Can you work these out from the model? Positions are in its coordinate system, mm. Coordinates: 2 decimals unless noted, no trailing zeros. Order: outer loops, then holes, each group sorted by start corner. A loop starts at its lowest first (then second) coordinate and runs counter-clockwise, first axis right, second up. Notation, with made-up numbers: (67.5, 32.25) -> (74.5, 32.25) arc R21 ccw to (74.5, 62.25) -> close; hole circle Ø4 at (87.25, 51). An arc over 180 degrees is marked (long way). Answer in a Markdown table with one row per item. Add a question column.
1. Imagine slicing it at D-D on y = 2.7. Write out the boundary of the cut face in (x, z), plus the area to 3 significant figures.
2. Imagine slicing it at B-B on x = -11.5. Write out the boundary of the cut face in (y, z), plus the area to 3 significant figures.
3. Imagine slicing it at C-C on x = -5. Write out the boundary of the cut face in (y, z), plus the area to 3 significant figures.
4. If I drill on line 1 along Z through (x, y) = (17.5, 2.6); line 2 along Z through (x, y) = (-9, 0.85); line 3 along Y through (x, z) = (9.5, 12.75), over which ranges is the centre line in solid material (lowest first)? Write a range as [from, to].
5. Imagine slicing it at A-A on y = 1.1. Write out the boundary of the cut face in (x, z), plus the area to 3 significant figures.
6. Will this pin go through, and if not, where does the flat tip stop? pin 1 (2 mm diameter, centred on x = -1.5, z = 3.5, fed in from -Y).
from build123d import *

# Parameters (mm, degrees)
F0_W        = 36.83
F0_H        = 3.048
F1_DEPTH    = 13.97
F3_T1_DEPTH = 60.1094845304
F4_DEPTH    = 25.4


# Not quite as in the source:
# - a fillet or chamfer that OpenCascade refuses, or shapes differently, is made with other operations: its cross-section is extruded or revolved along the edge and cut away or added


with BuildPart() as f1:
    # F0 (on Top) → F1 (new body)
    with BuildSketch(Plane.XY):
        with Locations((-0.254, 1.524)):
            Rectangle(F0_W, F0_H)
    extrude(amount=F1_DEPTH)

    # F3: fillet of radius 5.08 on 1 edges, made by hand

    # F3_s2 → F3_t1 (cut)
    with BuildSketch(Plane.YZ.offset(-30.3087422652)):
        with BuildLine():
            ThreePointArc((3.048, 9.3141030939), (2.2182329348, 12.0965336861), (0, 13.97))
            Line((0, 13.97), (3.048, 13.97))
            Line((3.048, 13.97), (3.048, 9.3141030939))
        make_face()
    extrude(amount=F3_T1_DEPTH, mode=Mode.SUBTRACT)

    # F2 (on face) → F4 (cut)
    with BuildSketch(Plane.XZ):
        Polygon((-15.494, 12.5322954744), (-14.6639409051, 13.97), (-16.3240590949, 13.97), align=None)
        Polygon((-4.3572939367, 13.97), (-6.3107060633, 13.97), (-5.334, 12.2782954744), align=None)
        Polygon((5.6560590949, 13.97), (3.9959409051, 13.97), (4.826, 12.5322954744), align=None)
        Polygon((15.8160590949, 13.97), (14.1559409051, 13.97), (14.986, 12.5322954744), align=None)
    extrude(amount=-F4_DEPTH, mode=Mode.SUBTRACT)


solid = f1.part
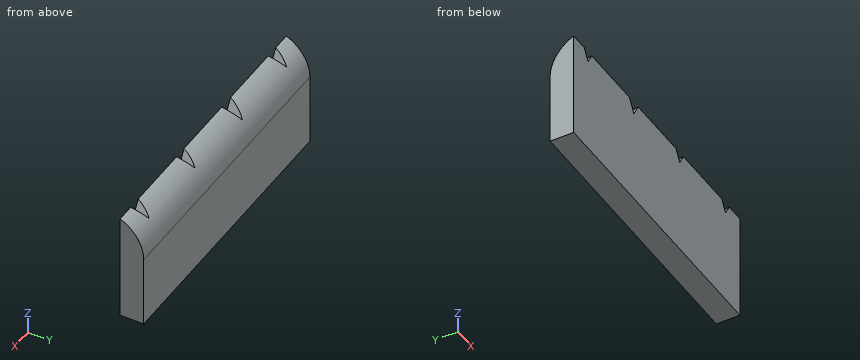
Answers follow:
| question | item | result |
|---|---|---|
| 1 | outline | (-18.67, 0) -> (18.16, 0) -> (18.16, 11.16) -> (-18.67, 11.16) -> close |
| 1 | area | 411 mm² |
| 2 | outline | (0, 0) -> (3.05, 0) -> (3.05, 9.31) arc R5.08 ccw to (0, 13.97) -> close |
| 2 | area | 38.6 mm² |
| 3 | outline | (0, 0) -> (3.05, 0) -> (3.05, 9.31) arc R5.08 ccw to (1.61, 12.86) -> (0, 12.86) -> close |
| 3 | area | 37.6 mm² |
| 4 | line 1 | z = [0, 11.4] |
| 4 | line 2 | z = [0, 13.5] |
| 4 | line 3 | y = [0, 1.71] |
| 5 | outline | (-18.67, 0) -> (18.16, 0) -> (18.16, 13.31) -> (15.44, 13.31) -> (14.99, 12.53) -> (14.53, 13.31) -> (5.28, 13.31) -> (4.83, 12.53) -> (4.37, 13.31) -> (-4.74, 13.31) -> (-5.33, 12.28) -> (-5.93, 13.31) -> (-15.04, 13.31) -> (-15.49, 12.53) -> (-15.95, 13.31) -> (-18.67, 13.31) -> close |
| 5 | area | 489 mm² |
| 6 | pin 1 | stops at y = 0 |
